Work out the finished part from the listing and answer in its coordinate system (mm). A direction names the side the tool comes from. Coordinates: 2 decimals unless noted, no trailing zeros. Write each loop counter-clockwise with the first axis right and the second up, starting at its lowest first coordinate (ties: lowest second). Pieces come first, ordered by that corner, then holes. Notation, with made-up numbers: (20.5, 81) -> (27.5, 81) arc R33 cw to (27.5, 119) -> close; hole circle Ø3 at (83, 43). An arc over 180 degrees is marked (long way). Write each question's results on one line, items separated by ' | '. Start each with the question number.
from build123d import *

# Parameters (mm, degrees)
F1_DEPTH = 152.4
F2_R     = 5.08
F3_R     = 6.35
F4_DEPTH = 106.681


with BuildPart() as f1:
    # F0 (on Front) → F1 (new body)
    with BuildSketch(Plane.XZ):
        Polygon((-46.99, -4.236735), (-46.99, 40.213265), (46.99, 40.213265), (46.99, -4.236735), (53.34, -4.236735), (53.34, 46.563265), (-53.34, 46.563265), (-53.34, -4.236735), align=None)
    extrude(amount=F1_DEPTH)

    # F2
    f2_edges = [f1.edges().sort_by_distance(p)[0] for p in [
        (-46.99, -76.2, 40.213265),
        (46.99, -76.2, 40.213265),
    ]]
    fillet(f2_edges, radius=F2_R)

    # F3 (on face) → F4 (cut, through all)
    with BuildSketch(Plane.YZ.offset(53.34)):
        with Locations((-133.35, 13.543265)):
            Circle(F3_R)
    extrude(amount=-F4_DEPTH, mode=Mode.SUBTRACT)


solid = f1.part
1. For faces 1 (the face through (0, -152.4, 42)), 2 (the face through (45.462, -77.267, 38.765)), determine the directions among +Z, -Z, +X, -X, +Y, -Y from which every point of the face is accessible in a straight line to the end or side of a thin tool.
2. Find section B-B on z = 27. Give the vertices of the cut face in (x, y), and give its area (3 significant figures).
3. Find the intervals of material crossed by L1, parallel to X at y = -112, z = 23; L2, parallel to Z at x = 50.5, y = -133.35; L3, parallel to Z at x = -40, y = -90.5, in increasing order.
4. Determine the mould class of faces 3 (the face through (-50, -75, -4.237)), 4 (the face through (-53.34, -75, 22)), 5 (the face through (-1, -75, 40.213)) for opening direction X: pulls with the +X half, pulls with the -X half, needs draft (parallel to the pull), parting line crosses it, or undercut.
5. Given pin 1 Ø10 at (y, z) = (-133.35, 13.54) entering from -X; pin 2 Ø5 at (x, y) = (19, -70) entering from -Z; pin 3 Ø16.5 at (y, z) = (-133.35, 13.54) entering from -X, each flat-ended and moving along its own axis, determine where each tip first touches the part or whether it passes through.
6. Find section C-C on z = 18. Give the vertices of the cut face in (x, y), and give its area (3 significant figures).
7. Find section A-A on y = -133.35. Give the vertices of the cut face in (x, z), and give its area (3 significant figures).
8. Find section D-D on x = 17.5. Give the vertices of the cut face in (y, z), and give its area (3 significant figures).
Ans:
1) face 1: +Z, -Z, +X, -X, -Y | face 2: -Z, +Y, -Y
2) outline: (-53.34, -152.4) -> (-46.99, -152.4) -> (-46.99, 0) -> (-53.34, 0) -> close; (46.99, -152.4) -> (53.34, -152.4) -> (53.34, 0) -> (46.99, 0) -> close | area: 1,940 mm²
3) L1: x = -53.34 to -46.99, 46.99 to 53.34 | L2: z = -4.24 to 7.19, 19.89 to 46.56 | L3: z = 40.21 to 46.56
4) face 3: needs draft | face 4: pulls with the -X half | face 5: undercut
5) pin 1: passes through | pin 2: stops at z = 40.21 | pin 3: stops at x = -53.34
6) outline: (-53.34, -152.4) -> (-46.99, -152.4) -> (-46.99, -137.87) -> (-53.34, -137.87) -> close; (-53.34, -128.83) -> (-46.99, -128.83) -> (-46.99, 0) -> (-53.34, 0) -> close; (46.99, -152.4) -> (53.34, -152.4) -> (53.34, -137.87) -> (46.99, -137.87) -> close; (46.99, -128.83) -> (53.34, -128.83) -> (53.34, 0) -> (46.99, 0) -> close | area: 1,820 mm²
7) outline: (-53.34, -4.24) -> (-46.99, -4.24) -> (-46.99, 7.19) -> (-53.34, 7.19) -> close; (-53.34, 19.89) -> (-46.99, 19.89) -> (-46.99, 35.13) arc R5.08 cw to (-41.91, 40.21) -> (41.91, 40.21) arc R5.08 cw to (46.99, 35.13) -> (46.99, 19.89) -> (53.34, 19.89) -> (53.34, 46.56) -> (-53.34, 46.56) -> close; (46.99, -4.24) -> (53.34, -4.24) -> (53.34, 7.19) -> (46.99, 7.19) -> close | area: 1,090 mm²
8) outline: (-152.4, 40.21) -> (0, 40.21) -> (0, 46.56) -> (-152.4, 46.56) -> close | area: 968 mm²
